from build123d import *

# Parameters (mm, degrees)
SKETCH_1_R      = 3
EXTRUDE_1_DEPTH = 2.6
SKETCH_2_R      = 2
EXTRUDE_2_DEPTH = 22.2
FILLET_1_R      = 0.5


with BuildPart() as part:
    # 草图1 → 凸台-拉伸1 (new body)
    with BuildSketch(Plane(origin=(0, 0, 0), x_dir=(1, 0, 0), z_dir=(0, 1, 0))):
        with Locations(Location((0, 0, 0), (0, 0, 270))):
            Circle(SKETCH_1_R)
    extrude(amount=EXTRUDE_1_DEPTH)

    # 草图2 → 凸台-拉伸2 (add)
    with BuildSketch(Plane(origin=(0, 2.6, 0), x_dir=(1, 0, 0), z_dir=(0, 1, 0))):
        with Locations(Location((0, 0, 0), (0, 0, 270))):
            Circle(SKETCH_2_R)
    extrude(amount=EXTRUDE_2_DEPTH)

    # 圆角1
    fillet_1_edges = [part.edges().sort_by_distance(p)[0] for p in [
        (0, 0, -3),
    ]]
    fillet(fillet_1_edges, radius=FILLET_1_R)


solid = part.part
CAD build for the part. Positions are in the model's coordinates, mm. Round coordinates to 2 decimals unless told otherwise and drop trailing zeros. Loops run counter-clockwise (first coordinate to the right, second up) from the corner with the lowest first, then second, coordinate; pieces in that order, holes last.
(1) Cut at B-B (x = 0). Give the cut face in (y, z), plus the area to 3 significant figures.
(2) Cut at C-C (y = 14). Give the cut face in (x, z).
(3) Cut at A-A (z = 0). Give the cut face in (x, y).
(4) Drop flat-ended pins along their axis: pin 1 (1.5 mm diameter, centred on x = -1.5, y = 21, fed in from +Z); pin 2 (1 mm diameter, centred on x = 2, z = -2, fed in from -Y); pin 3 (1.5 mm diameter, centred on x = -1.5, y = 15, fed in from -Z); pin 4 (3 mm diameter, centred on y = 7.5, z = 1, fed in from +X). Give the stop position or say it passes through.
(5) Two-plate mould, pull along Y, no slides. Class faces 1 (the flat face through (-1, 2.6, 2)), 2 (the flat face through (0, 0, 0)), 3 (the cylindrical face through (-2, 14, 0)): +Y half, -Y half, draft (parallel to the pull), parting line (faces both ways), or undercut.
(6) Wall check: line 1 along Y through (x, z) = (0.65, 2); line 2 along X through (y, z) = (3.25, 0); line 3 along X through (y, z) = (23.5, 1.5). Give the ranges that are in metal, low to high.
Findings below:
1. outline: (0, -2.5) arc R0.5 ccw to (0.5, -3) - (2.6, -3) - (2.6, -2) - (24.8, -2) - (24.8, 2) - (2.6, 2) - (2.6, 3) - (0.5, 3) arc R0.5 ccw to (0, 2.5) - close
1. area: 104 mm2
2. outline: circle Ø4 at (0, 0)
3. outline: (-3, 0.5) arc R0.5 ccw to (-2.5, 0) - (2.5, 0) arc R0.5 ccw to (3, 0.5) - (3, 2.6) - (2, 2.6) - (2, 24.8) - (-2, 24.8) - (-2, 2.6) - (-3, 2.6) - close
4. pin 1: stops at z = 1.85
4. pin 2: stops at y = 0
4. pin 3: stops at z = -1.85
4. pin 4: stops at x = 2
5. face 1: +Y half
5. face 2: -Y half
5. face 3: draft
6. line 1: y = 0 to 2.6
6. line 2: x = -2 to 2
6. line 3: x = -1.32 to 1.32
